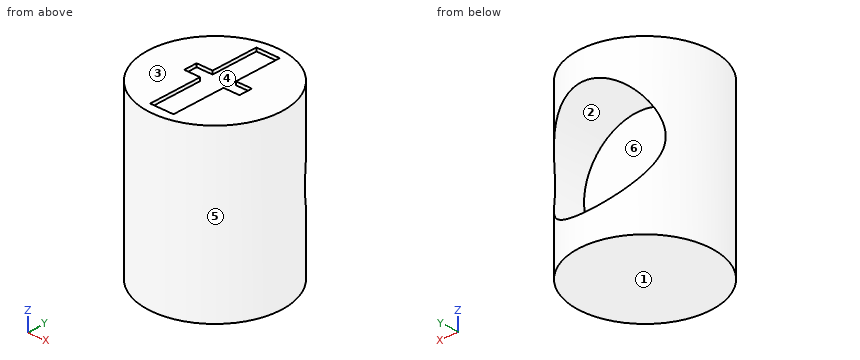
from build123d import *

# Parameters (mm, degrees)
CROQUIS1_R                = 20
SALIENTE_EXTRUIR1_DEPTH   = 50
CORTAR_EXTRUIR2_START     = 7.820318539
CORTAR_EXTRUIR2_OUTLINE_R = 16.6
CORTAR_EXTRUIR2_DEPTH     = 12.179681561
CORTAR_EXTRUIR4_DEPTH     = 1
CORTAR_EXTRUIR5_START     = -6
CROQUIS10_R               = 16.6
CORTAR_EXTRUIR5_DEPTH     = 6


# Read off the part's stored shape, not the designer's step: Cortar-Extruir2
with BuildPart() as part:
    # Croquis1 → Saliente-Extruir1 (new body)
    with BuildSketch(Plane.XY):
        Circle(CROQUIS1_R)
    extrude(amount=SALIENTE_EXTRUIR1_DEPTH)

    # Cortar-Extruir2 outline → Cortar-Extruir2 (cut)
    with BuildSketch(Plane(origin=(0, 0, 0), x_dir=(1, 0, 0), z_dir=(0, 1, 0)).offset(CORTAR_EXTRUIR2_START)):
        with Locations((0, -25)):
            Circle(CORTAR_EXTRUIR2_OUTLINE_R)
    extrude(amount=CORTAR_EXTRUIR2_DEPTH, mode=Mode.SUBTRACT)

    # Croquis4 → Cortar-Extruir4 (cut)
    with BuildSketch(Plane.XY.offset(50)):
        Polygon((8.3, 3), (3.5, 3), (3.5, 17.1), (-3.5, 17.1), (-3.5, 3), (-8.3, 3), (-8.3, 1), (-8.3, -1), (-3.5, -1), (-3.5, -2), (-3.5, -17.1), (3.5, -17.1), (3.5, -2), (3.5, -1), (8.3, -1), (8.3, 1), align=None)
    extrude(amount=-CORTAR_EXTRUIR4_DEPTH, mode=Mode.SUBTRACT)

    # Croquis10 → Cortar-Extruir5 (cut)
    with BuildSketch(Plane(origin=(0, 7.820318539, 0), x_dir=(1, 0, 0), z_dir=(0, 1, 0)).offset(CORTAR_EXTRUIR5_START)):
        with Locations(Location((0, -25, 0), (0, 0, 90))):
            Circle(CROQUIS10_R)
    extrude(amount=CORTAR_EXTRUIR5_DEPTH, mode=Mode.SUBTRACT)


solid = part.part
Read the model definition and answer for the solid it produces. Units are mm, in the model's axes. Face numbers are marked on the shaded views. A direction names the side the tool comes from. Round coordinates to 2 decimals unless told otherwise and drop trailing zeros. Loops run counter-clockwise (first coordinate to the right, second up) from the corner with the lowest first, then second, coordinate; pieces in that order, holes last. Notation, with made-up numbers: (-22, -23.5) - (-5, -23.5) arc R13 cw to (-5, -13.5) - close; hole circle Ø8 at (52, 53.5). An arc over 180 degrees is marked (long way). One line per question, with ' | ' between items. Start each with the question number.
Q1. Section A-A on x = 0 is taken. Give the vertices of the cut face in (y, z), plus the area to 3 significant figures.
Q2. Section B-B on y = 5.5 is taken. Give the vertices of the cut face in (x, z), plus the area to 3 significant figures.
Q3. For a pull along Y with two mould halves and no side action, classify the marked faces 3, 4, 5 and 6 as +Y half, -Y half, draft (parallel to the pull), parting line (faces both ways), or undercut.
Q4. Section D-D on y = -14 is taken. Give the vertices of the cut face in (x, z), plus the area to 3 significant figures.
Q5. Flat-ended cylindrical pins translate along their axes: pin 1 (0.8 mm diameter, centred on x = -5, z = 49.5, fed in from -Y); pin 2 (0.5 mm diameter, centred on y = 12, z = 49.5, fed in from -X); pin 3 (5 mm diameter, centred on y = -12, z = 24.5, fed in from -X). Find the tip coordinate at first contact, or state that the pin passes through.
Q6. For the marked faces 1 and 2, determine the directions among +Z, -Z, +X, -X, +Y, -Y from which every point of the face is accessible in a straight line to the end or side of a thin tool.
Q7. Find the intervals of material crossed by L1, parallel to Z at x = 0, y = 13.5; L2, parallel to X at y = 2.5, z = 11.5; L3, parallel to Y at x = -14.5, z = 32, in increasing order.
Q8. Section C-C on z = 44.5 is taken. Give the vertices of the cut face in (x, y).
Established:
1) outline: (-20, 0) - (20, 0) - (20, 8.4) - (1.82, 8.4) - (1.82, 41.6) - (20, 41.6) - (20, 50) - (17.1, 50) - (17.1, 49) - (-17.1, 49) - (-17.1, 50) - (-20, 50) - close | area: 1,360 mm²
2) outline: (-19.23, 0) - (19.23, 0) - (19.23, 50) - (3.5, 50) - (3.5, 49) - (-3.5, 49) - (-3.5, 50) - (-19.23, 50) - close; hole circle Ø33.2 at (0, 25) | area: 1,050 mm²
3) face 3: draft | face 4: undercut | face 5: parting line | face 6: +Y half
4) outline: (-14.28, 0) - (14.28, 0) - (14.28, 50) - (3.5, 50) - (3.5, 49) - (-3.5, 49) - (-3.5, 50) - (-14.28, 50) - close | area: 1,420 mm²
5) pin 1: y = -19.46 | pin 2: x = -16.18 | pin 3: x = -17.6
6) face 1: -Z, +X, -X, +Y, -Y | face 2: +Y
7) L1: 0 to 8.4, 41.6 to 49 | L2: -19.84 to -9.66, 9.66 to 19.84 | L3: -13.77 to 1.82
8) outline: circle Ø40 at (0, 0)
